Part model, mm, in its own coordinate system. A direction names the side the tool comes from. Give positions to 0.01 mm unless a question says otherwise; leave off trailing zeros. Order: outer loops, then holes, each group sorted by start corner. A loop starts at its lowest first (then second) coordinate and runs counter-clockwise, first axis right, second up. Notation, with made-up numbers: M 55.25,11 L 90.25,11 A18 cw 90.25,26 Z; hole C 69.25,32 d1. An arc over 180 degrees is marked long. One line per question, with ' | ' between items.
Autodesk Inventor part; units mm, degrees
ref_plane "YZ Plane" through (0, 0, 0) normal (1, 0, 0) x (0, 1, 0)
ref_plane "XZ Plane" through (0, 0, 0) normal (0, 1, 0) x (-1, 0, 0)
ref_plane "XY Plane" through (0, 0, 0) normal (0, 0, 1) x (1, 0, 0)
sketch "Boceto1" plane through (0, 0, 0) normal (0, 0, 1) x (1, 0, 0)
  line L0 (0, 0) -> (30, 0)
  line L1 (30, 0) -> (30, 30)
  line L2 (30, 30) -> (0, 30)
  line L3 (0, 30) -> (0, 0)
  circle A0 centre (15, 15) radius 4
  circle A1 centre (15, 23.5) radius 1.5
  circle A2 centre (15, 6.5) radius 1.5
  dimension "d0" = 30
  dimension "d1" = 30
  dimension "d2" = 8
  dimension "d3" = 3
  dimension "d4" = 3
  dimension "d5" = 8.5
  dimension "d6" = 8.5
  dimension "d7" = 6.5
extrude "Extrusión1" add sketch "Boceto1" along normal blind 5
sketch "Boceto2" plane through (0, 0, 0) normal (0, 0, -1) x (-1, 0, 0)
  line L0 (-30, 0) -> (-30, 30)
  line L1 (-30, 0) -> (0, 0)
  line L2 (0, 0) -> (0, -5)
  line L3 (0, -5) -> (-30, -5)
  line L4 (-30, -5) -> (-30, 0)
  dimension "d10" = 5
extrude "Extrusión2" add sketch "Boceto2" against normal blind 35
sketch "Boceto3" plane through (0, 0, 5) normal (0, 1, 0) x (1, 0, 0)
  line L0 (6.75, -8.25) -> (6.75, -23.25) construction
  line L1 (5, -8.25) -> (5, -23.25)
  line L2 (8.5, -23.25) -> (8.5, -8.25)
  arc A0 (8.5, -8.25) -> (5, -8.25) centre (6.75, -8.25) ccw
  arc A1 (5, -23.25) -> (8.5, -23.25) centre (6.75, -23.25) ccw
  line L3 (23.25, -8.25) -> (23.25, -23.25) construction
  line L4 (21.5, -8.25) -> (21.5, -23.25)
  line L5 (25, -23.25) -> (25, -8.25)
  arc A2 (25, -8.25) -> (21.5, -8.25) centre (23.25, -8.25) ccw
  arc A3 (21.5, -23.25) -> (25, -23.25) centre (23.25, -23.25) ccw
  line L6 (0, 0) -> (0, -30)
  line L7 (30, 0) -> (30, -30)
  line L8 (30, -30) -> (0, -30)
  point P0 (0, 5)
  point P1 (6.75, -15.75)
  point P2 (23.25, -15.75)
  point P3 (6.75, -25)
  dimension "d13" = 3.5
  dimension "d14" = 3.5
  dimension "d15" = 15
  dimension "d16" = 15
  dimension "d17" = 5
  dimension "d18" = 5
  dimension "d19" = 0
  dimension "d20" = 5
extrude "Extrusión3" cut sketch "Boceto3" against normal blind 5
fillet "Empalme1" radius 2 1 edges at (15, -5, 0)
fillet "Empalme2" radius 2 5 edges at (0, -2.5, 35) (30, -2.5, 35) (30, 30, 2.5) (0, 30, 2.5) (15, 0, 5)
properties part number "soporte_motor"
1. Slice it at A-A on y = 23.5. Give the cut face in (x, z), then the cut area to 3 significant figures.
Worked out:
outline: M 0,0 L 13.5,0 L 13.5,5 L 0,5 Z; M 16.5,0 L 30,0 L 30,5 L 16.5,5 Z | area: 135 mm2
2. Slice it at B-B on x = 15. Give the cut face in (y, z).
Worked out:
outline: M -5,2 A2 ccw -3,0 L 5,0 L 5,5 L 2,5 A2 cw 0,7 L 0,35 L -5,35 Z; M 8,0 L 11,0 L 11,5 L 8,5 Z; M 19,0 L 22,0 L 22,5 L 19,5 Z; M 25,0 L 30,0 L 30,5 L 25,5 Z
3. Slice it at D-D on x = 23.25. Give the cut face in (y, z), then the cut area to 4 significant figures.
Worked out:
outline: M -5,2 A2 ccw -3,0 L 30,0 L 30,5 L 2,5 A2 cw 0,7 L 0,11.5 L -5,11.5 Z; M -5,30 L 0,30 L 0,35 L -5,35 Z | area: 232.5 mm2
4. Slice it at C-C on z = 24.5. Give the cut face in (x, y).
Worked out:
outline: M 0,-5 L 5,-5 L 5,0 L 0,0 Z; M 8.5,-5 L 21.5,-5 L 21.5,0 L 8.5,0 Z; M 25,-5 L 30,-5 L 30,0 L 25,0 Z
5. Mould opens along Y. For faces 1 (the cylindrical face through (23.3, -2.5, 11.5)), 2 (the cylindrical face through (13.89, 22.49, 2.46)), 3 (the cylindrical face through (15.21, -4.43, 0.6)) say: released by +Y, released by -Y, zero draft, split by the parting line, or undercut.
Worked out:
face 1: zero draft | face 2: undercut | face 3: released by -Y
6. Tool access for faces 4 (the cylindrical face through (6.8, -2.5, 11.5)), 5 (the flat face through (30, -1, 10)), 6 (the flat face through (14.8, 19.3, 5)): list every direction of +Z, -Z, +X, -X, +Y, -Y with a clear straight run to the whole face (end or side of a thin tool).
Worked out:
face 4: +Y, -Y | face 5: +Z, -Z, +X, +Y, -Y | face 6: +Z, +X, -X, +Y
7. Probe L1, parallel to Y at x = 15, z = 4.05; L2, parallel to Y at x = 15, z = 1.4; L3, parallel to Z at x = 12, y = 29. List the from-to ranges inside material, lowest first. Write a range as from..to.
Worked out:
L1: y = -5..5, 8..11, 19..22, 25..30 | L2: y = -4.91..5, 8..11, 19..22, 25..30 | L3: z = 0..5
8. Drop flat-ended pins along their axis: pin 1 (12 mm diameter, centred on x = 22.5, z = 13.5, fed in from -Y); pin 2 (2.5 mm diameter, centred on x = 15, y = 23.5, fed in from -Z); pin 3 (14 mm diameter, centred on x = 11.5, z = 22, fed in from +Y); pin 4 (10.5 mm diameter, centred on x = 15, y = 15, fed in from +Z). Give the stop position or say it passes through.
Worked out:
pin 1: stops at y = -5 | pin 2: passes through | pin 3: stops at y = 0 | pin 4: stops at z = 5
